Geometry check sheet. Reference: the model listing, model coordinates, mm. A direction names the side the tool comes from. Give positions to 0.01 mm unless a question says otherwise; leave off trailing zeros. Write each loop counter-clockwise with the first axis right and the second up, starting at its lowest first coordinate (ties: lowest second). Pieces come first, ordered by that corner, then holes. Notation, with made-up numbers: (-6.5, 70.25) -> (24.5, 70.25) arc R22 cw to (24.5, 94.25) -> close; hole circle Ø10 at (-28, -2.5). An arc over 180 degrees is marked (long way). Use a Markdown table: item, result. Add a question column.
from build123d import *

# Parameters (mm, degrees)
BOSS_EXTRUDE1_REACH      = 46.947
BOSS_EXTRUDE1_END_RADIUS = 6.2
SKETCH2_R                = 1.45


with BuildPart() as part:
    # Sketch1 → Revolve1 (revolve)
    with BuildSketch(Plane(origin=(0, 0, 0), x_dir=(-1, 0, 0), z_dir=(0, 0, -1)), mode=Mode.PRIVATE) as revolve1_sk:
        with BuildLine():
            Line((-30, 1.5), (-30, 0))
            Line((-30, 0), (0, 0))
            ThreePointArc((0, 0), (-0.439339828, 1.060660172), (-1.5, 1.5))
            Line((-1.5, 1.5), (-24.5, 1.5))
            ThreePointArc((-24.5, 1.5), (-25, 1), (-25.5, 1.5))
            Line((-25.5, 1.5), (-30, 1.5))
        make_face()
    revolve(revolve1_sk.sketch.rotate(Axis((30, 0, 0), (-1, 0, 0)), 270), axis=Axis((30, 0, 0), (-1, 0, 0)))

    # Boss-Extrude1: up to this cylinder (the profile starts outside it)
    boss_extrude1_end = Plane(origin=(82, 0, 0), z_dir=(0, 0.7071067811865475, 0.7071067811865476)) * Cylinder(BOSS_EXTRUDE1_END_RADIUS, 107.294, mode=Mode.PRIVATE)
    # Sketch2 → Boss-Extrude1 (add, up to the surface)
    with BuildSketch(Plane(origin=(30, 0, 0), x_dir=(0, 0, -1), z_dir=(1, 0, 0)), mode=Mode.PRIVATE) as boss_extrude1_sk1:
        with Locations(Location((0, 0, 0), (0, 0, 180.053796912))):
            Circle(SKETCH2_R)
    boss_extrude1_tool1 = extrude(boss_extrude1_sk1.sketch, amount=BOSS_EXTRUDE1_REACH, mode=Mode.PRIVATE) - boss_extrude1_end
    add(boss_extrude1_tool1.solids().sort_by_distance((30, 0, 0))[0])


solid = part.part
1) Material ranges on probe 1 along Y at (x, z) = (56.5, 0.15); probe 2 along Z at (x, y) = (4, -0.1); probe 3 along X at (y, z) = (0, 1.1), recorded low to high. Write a range as [from, to].
2) Sectioned sample at B-B, the plane x = 46.5. Enter the section's corners in (y, z), and give its area (3 significant figures).
3) Sectioned sample at A-A, the plane x = 8. Enter the section's corners in (y, z).
4) Draft check along Y on faces 3 (the face through (13.16, 0.45, 1.43)), 4 (the face through (75.8, 0, 0)). Enter one of: +Y half, -Y half, draft (parallel to the pull), parting line (faces both ways), or undercut.
5) Gauge pin test, flat end, axial feed: P1, Ø1, axis at x = 28.5, y = 1, coming from the -Z side. Record the tip position at first contact, or that the pin passes through.
6) Tool access check on faces 1 (the face through (27.78, 0.45, 1.43)), 2 (the face through (52.66, -0.44, 1.38)). Record the directions out of +Z, -Z, +X, -X, +Y, -Y that give a thin tool (end or side, any length) a straight path to the whole face; none if there is none.
Check values:
| question | item | result |
|---|---|---|
| 1 | probe 1 | [-1.44, 1.44] |
| 1 | probe 2 | [-1.5, 1.5] |
| 1 | probe 3 | [0.48, 24.7], [25.3, 75.85] |
| 2 | outline | circle Ø2.9 at (0, 0) |
| 2 | area | 6.61 mm² |
| 3 | outline | circle Ø3 at (0, 0) |
| 4 | face 3 | parting line |
| 4 | face 4 | undercut |
| 5 | P1 | z = -1.41 |
| 6 | face 1 | +X, -X |
| 6 | face 2 | +X |
